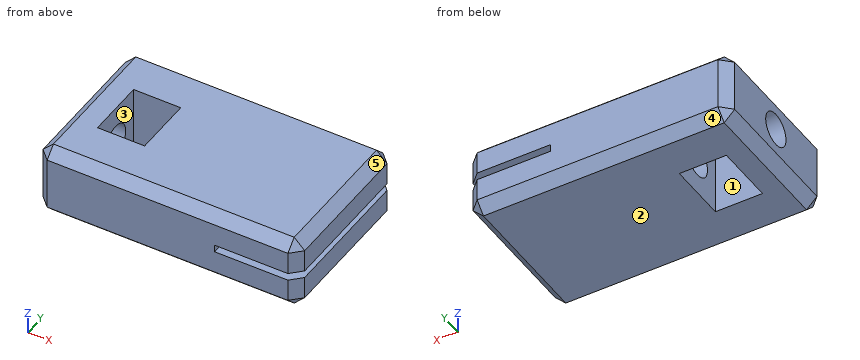
```python
from build123d import *

# Parameters (mm, degrees)
BOSS_EXTRUDE1_DEPTH = 7.5
SKETCH3_R           = 1.6
CUT_EXTRUDE1_DEPTH  = 16
SKETCH4_W           = 4.5
SKETCH4_H           = 5.7
CUT_EXTRUDE2_DEPTH  = 28.023138234
CHAMFER1_SIZE       = 1


with BuildPart() as part:
    # Sketch2 → Boss-Extrude1 (new, symmetric)
    with BuildSketch(Plane(origin=(0, 0, 0), x_dir=(1, 0, 0), z_dir=(0, 1, 0))):
        Polygon((25, -0.35), (25, -3.5), (0, -3.5), (0, 3.5), (25, 3.5), (25, 0.35), (17, 0.35), (17, -0.35), align=None)
    extrude(amount=BOSS_EXTRUDE1_DEPTH, both=True)

    # Sketch3 → Cut-Extrude1 (cut)
    with BuildSketch(Plane.ZY):
        Circle(SKETCH3_R)
    extrude(amount=-CUT_EXTRUDE1_DEPTH, mode=Mode.SUBTRACT)

    # Sketch4 → Cut-Extrude2 (cut, through all)
    with BuildSketch(Plane.XY.offset(3.5)):
        with Locations((5.25, 0)):
            Rectangle(SKETCH4_W, SKETCH4_H)
    extrude(amount=-CUT_EXTRUDE2_DEPTH, mode=Mode.SUBTRACT)

    # Chamfer1
    chamfer1_edges = [part.edges().sort_by_distance(p)[0] for p in [
        (25, 7.5, 1.925),
        (12.5, -7.5, 3.5),
        (0, -7.5, 0),
        (0, 0, -3.5),
        (25, 0, -3.5),
        (25, 0, 3.5),
        (0, 0, 3.5),
        (25, 7.5, -1.925),
        (12.5, 7.5, -3.5),
        (0, 7.5, 0),
        (12.5, 7.5, 3.5),
        (12.5, -7.5, -3.5),
        (25, -7.5, -1.925),
        (25, -7.5, 1.925),
    ]]
    chamfer(chamfer1_edges, length=CHAMFER1_SIZE)


solid = part.part
```
Verification items for the finished model (mm, model axes). Face numbers are marked on the shaded views. A direction names the side the tool comes from. Coordinates: 2 decimals unless noted, no trailing zeros. Order: outer loops, then holes, each group sorted by start corner. A loop starts at its lowest first (then second) coordinate and runs counter-clockwise, first axis right, second up. Notation, with made-up numbers: (34.25, -11.5) -> (54.25, -11.5) arc R13 cw to (54.25, 1.5) -> close; hole circle Ø1 at (68, -13.5). An arc over 180 degrees is marked (long way). Put each result on its own line as item: value. Start each with the question number.
1) Cross-section at B-B (z = -2). Enter the section's corners in (x, y).
2) Go/stop test with flat-tipped pins: pin 1 (1.7 mm diameter, centred on y = -0.5, z = 0, fed in from -X); pin 2 (2.5 mm diameter, centred on y = 0.5, z = 0, fed in from -X). Record where each tip stops, or that it passes through.
3) Tool access check on the marked faces 1 and 2. Record the directions out of +Z, -Z, +X, -X, +Y, -Y that give a thin tool (end or side, any length) a straight path to the whole face; none if there is none.
4) Cross-section at A-A (y = 0). Enter the section's corners in (x, z).
5) Material ranges on L1, parallel to Y at x = 1.4, z = 0; L2, parallel to Z at x = 19, y = 3.5; L3, parallel to X at y = -1.5, z = 1.25, recorded low to high.
6) Cross-section at D-D (y = -4). Enter the section's corners in (x, z).
7) Release check for a two-part mould opening along X. For the marked faces 3, 4 and 5 record: pulls with the +X half, pulls with the -X half, needs draft (parallel to the pull), parting line crosses it, or undercut.
8) Cross-section at C-C (x = 4). Enter the section's corners in (y, z), plus the area to 3 significant figures.
Geometry check:
1. outline: (0, -6.5) -> (1, -7.5) -> (24, -7.5) -> (25, -6.5) -> (25, 6.5) -> (24, 7.5) -> (1, 7.5) -> (0, 6.5) -> close; hole (3, -2.85) -> (7.5, -2.85) -> (7.5, 2.85) -> (3, 2.85) -> close
2. pin 1: stops at x = 16
2. pin 2: stops at x = 0
3. face 1: +Z, -Z
3. face 2: -Z, +X, -X, +Y, -Y
4. outline: (0, -2.5) -> (1, -3.5) -> (3, -3.5) -> (3, -1.6) -> (0, -1.6) -> close; (0, 1.6) -> (3, 1.6) -> (3, 3.5) -> (1, 3.5) -> (0, 2.5) -> close; (7.5, -3.5) -> (24, -3.5) -> (25, -2.5) -> (25, -0.35) -> (17, -0.35) -> (17, 0.35) -> (25, 0.35) -> (25, 2.5) -> (24, 3.5) -> (7.5, 3.5) -> (7.5, 1.6) -> (16, 1.6) -> (16, -1.6) -> (7.5, -1.6) -> close
5. L1: y = -7.5 to -1.6, 1.6 to 7.5
5. L2: z = -3.5 to -0.35, 0.35 to 3.5
5. L3: x = 0 to 3, 7.5 to 25
6. outline: (0, -2.5) -> (1, -3.5) -> (24, -3.5) -> (25, -2.5) -> (25, -0.35) -> (17, -0.35) -> (17, 0.35) -> (25, 0.35) -> (25, 2.5) -> (24, 3.5) -> (1, 3.5) -> (0, 2.5) -> close
7. face 3: undercut
7. face 4: needs draft
7. face 5: pulls with the +X half
8. outline: (-7.5, -2.5) -> (-6.5, -3.5) -> (-2.85, -3.5) -> (-2.85, 3.5) -> (-6.5, 3.5) -> (-7.5, 2.5) -> close; (2.85, -3.5) -> (6.5, -3.5) -> (7.5, -2.5) -> (7.5, 2.5) -> (6.5, 3.5) -> (2.85, 3.5) -> close
8. area: 63.1 mm^2
